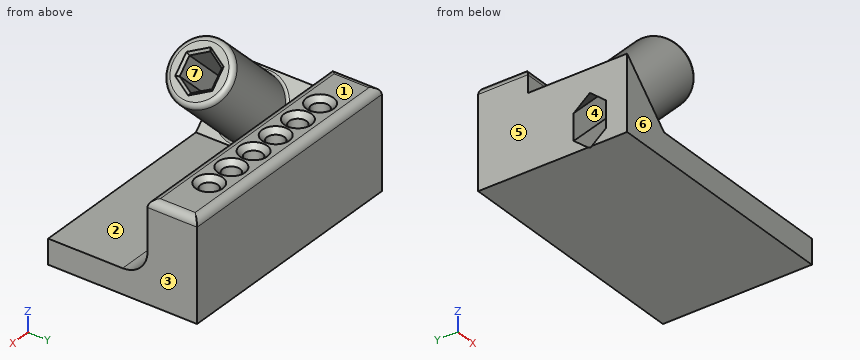
from build123d import *

# Parameters (mm, degrees)
SKETCH_W            = 100
SKETCH_H            = 60
PAD_DEPTH           = 10
SKETCH001_W         = 100
SKETCH001_H         = 20
PAD001_DEPTH        = 30
SKETCH002_R         = 3.5
POCKET_DEPTH        = 30
LINEARPATTERN_COUNT = 6
LINEARPATTERN_PITCH = 12
CHAMFER_SIZE        = 2
FILLET_R            = 10
FILLET001_R         = 3
PAD002_DEPTH        = 60
SKETCH004_R         = 12.5
PAD003_DEPTH        = 40
POCKET001_DEPTH     = 61.2142034356
FILLET002_R         = 2
CHAMFER001_SIZE     = 1
FILLET003_R         = 1


with BuildPart() as part:
    # Sketch → Pad (new body)
    with BuildSketch(Plane.XY):
        with Locations((50, 30)):
            Rectangle(SKETCH_W, SKETCH_H)
    extrude(amount=PAD_DEPTH)

    # Sketch001 (on Face6 of Pad) → Pad001 (join)
    with BuildSketch(Plane.XY.offset(10)):
        with Locations((50, 50)):
            Rectangle(SKETCH001_W, SKETCH001_H)
    extrude(amount=PAD001_DEPTH)

    # Sketch002 (on Face11 of Pad001) → Pocket (cut)
    with BuildSketch(Plane.XY.offset(40)):
        with Locations((80, 50)):
            Circle(SKETCH002_R)
    pocket = extrude(amount=-POCKET_DEPTH, mode=Mode.SUBTRACT)

    # LinearPattern: Pocket ×6
    with Locations(*[(-i * LINEARPATTERN_PITCH, 0, 0) for i in range(1, LINEARPATTERN_COUNT)]):
        add(pocket, mode=Mode.SUBTRACT)

    # Chamfer
    chamfer_edges = [part.edges().sort_by_distance(p)[0] for p in [
        (28.5, 50, 40),
        (16.5, 50, 40),
        (40.5, 50, 40),
        (52.5, 50, 40),
        (64.5, 50, 40),
        (76.5, 50, 40),
    ]]
    chamfer(chamfer_edges, length=CHAMFER_SIZE)

    # Fillet
    fillet_edges = [part.edges().sort_by_distance(p)[0] for p in [
        (50, 40, 10),
    ]]
    fillet(fillet_edges, radius=FILLET_R)

    # Fillet001
    fillet001_edges = [part.edges().sort_by_distance(p)[0] for p in [
        (0, 50, 40),
        (50, 60, 40),
        (50, 40, 40),
        (100, 50, 40),
    ]]
    fillet(fillet001_edges, radius=FILLET001_R)

    # Sketch003 (on Face13 of Fillet001) → Pad002 (join)
    with BuildSketch(Plane.XZ):
        Polygon((0, 10), (0, 30), (20, 10), align=None)
    extrude(amount=-PAD002_DEPTH)

    # Sketch004 (on Face7 of Pad002) → Pad003 (join)
    with BuildSketch(Plane(origin=(15, 0, 15), x_dir=(0, 1, 0), z_dir=(0.7071067812, 0, 0.7071067812))):
        with Locations((15, 7.0710678119)):
            Circle(SKETCH004_R)
    extrude(amount=PAD003_DEPTH)

    # Sketch005 (on Face22 of Pad003) → Pocket001 (cut, through all)
    with BuildSketch(Plane(origin=(43.2842712475, 0, 43.2842712475), x_dir=(0.7071067812, 0, -0.7071067812), z_dir=(0.7071067812, 0, 0.7071067812))):
        Polygon((-3.3182910621, 21.5), (-10.8238445616, 21.5), (-14.5766213113, 15), (-10.8238445616, 8.5), (-3.3182910621, 8.5), (0.4344856876, 15), align=None)
    extrude(amount=-POCKET001_DEPTH, mode=Mode.SUBTRACT)

    # Fillet002
    fillet002_edges = [part.edges().sort_by_distance(p)[0] for p in [
        (38.284271, 2.5, 48.284271),
    ]]
    fillet(fillet002_edges, radius=FILLET002_R)

    # Chamfer001
    chamfer001_edges = [part.edges().sort_by_distance(p)[0] for p in [
        (38.284271, 21.5, 48.284271),
        (34.30385, 18.25, 52.264692),
        (34.30385, 11.75, 52.264692),
        (38.284271, 8.5, 48.284271),
        (42.264692, 11.75, 44.30385),
        (42.264692, 18.25, 44.30385),
    ]]
    chamfer(chamfer001_edges, length=CHAMFER001_SIZE)

    # Fillet003
    fillet003_edges = [part.edges().sort_by_distance(p)[0] for p in [
        (10, 2.5, 20),
    ]]
    fillet(fillet003_edges, radius=FILLET003_R)


solid = part.part
Model file for the job. Use its own axes, mm. Face numbers are marked on the shaded views. A direction names the side the tool comes from. Coordinates: 2 decimals unless noted, no trailing zeros. Write each loop counter-clockwise with the first axis right and the second up, starting at its lowest first coordinate (ties: lowest second). Pieces come first, ordered by that corner, then holes. Notation, with made-up numbers: (67.25, 12.25) - (119.25, 12.25) arc R14 ccw to (119.25, 34.25) - close; hole circle Ø5 at (-26, -19). An arc over 180 degrees is marked (long way). Write each question's results on one line, items separated by ' | '. Start each with the question number.
1) Cut at D-D (x = 92). Write the cut outline in (y, z).
2) Cut at C-C (z = 25.5). Count the separate pieces of the cut face and the enclosed holes in it, then the cut area to 3 significant figures.
3) 3-axis set-ups, long thin cutter, end or side, ignore diameter. For the marked faces 1, 2 and 3: which of +Z, -Z, +X, -X, +Y, -Y reach the whole face in a straight line?
4) Cut at A-A (x = 80). Write the cut outline in (y, z), then the cut area to 3 significant figures.
5) Probe line 1 along Y through (x, z) = (32, 26); line 2 along Y through (x, z) = (56, 28.25); line 3 along Y through (x, z) = (32, 28.75). List the from-to ranges inside material, lowest first. Write a range as from..to.
6) Cut at B-B (y = 38). Write the cut outline in (x, z).
7) Flat gauge pins, fed straight in: P1, Ø3, axis at x = 25, y = 20.5, coming from the +Z side; P2, Ø8, axis at x = 32, y = 50, coming from the +Z side; P3, Ø6, axis at y = 24, z = 49.5, coming from the -X side. Where does each tip first touch, or does it go through?
8) Mould opens along X. For the marked faces 4, 5, 6 and 7 say: pulls with the +X half, pulls with the -X half, needs draft (parallel to the pull), parting line crosses it, or undercut.
Returned:
1) outline: (0, 0) - (60, 0) - (60, 37) arc R3 ccw to (57, 40) - (43, 40) arc R3 ccw to (40, 37) - (40, 20) arc R10 cw to (30, 10) - (0, 10) - close
2) separate pieces: 1 | enclosed holes: 7 | area: 2,350 mm^2
3) face 1: +Z, +X, -X, +Y | face 2: +X, -Y | face 3: +Z, -Z, +X, +Y, -Y
4) outline: (0, 0) - (60, 0) - (60, 37) arc R3 ccw to (57, 40) - (55.5, 40) - (53.5, 38) - (53.5, 10) - (46.5, 10) - (46.5, 38) - (44.5, 40) - (43, 40) arc R3 ccw to (40, 37) - (40, 20) arc R10 cw to (30, 10) - (0, 10) - close | area: 1,000 mm^2
5) line 1: 9.68..20.32, 40..46.5, 53.5..60 | line 2: 40..46.5, 53.5..60 | line 3: 6.73..23.27, 40..46.5, 53.5..60
6) outline: (0, 0) - (100, 0) - (100, 14) - (16, 14) - (0, 30) - close
7) P1: z = 52.65 | P2: z = 38.5 | P3: x = 22.62
8) face 4: undercut | face 5: pulls with the -X half | face 6: needs draft | face 7: undercut
